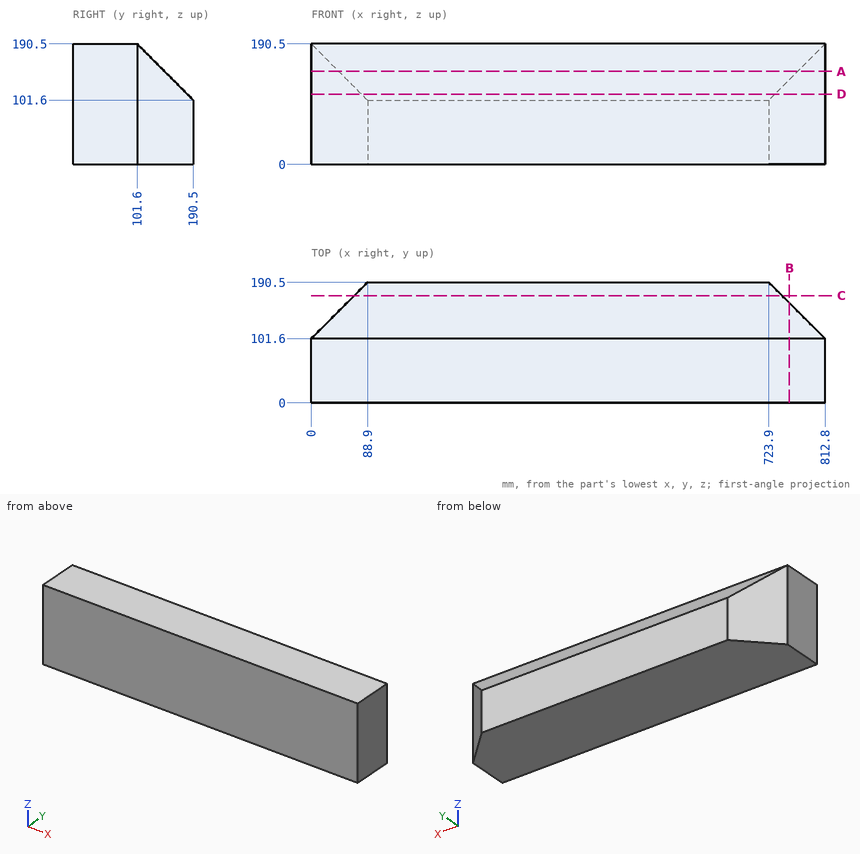
Source: three-view drawing plus pictorial views. Frame: mm from the lowest corner of the part. Round coordinates to 2 decimals unless told otherwise and drop trailing zeros. Loops run counter-clockwise (first coordinate to the right, second up) from the corner with the lowest first, then second, coordinate; pieces in that order, holes last. Notation, with made-up numbers: (-26.75, -20) - (20.25, -20) arc R19 ccw to (20.25, 1) - close; hole circle Ø5 at (81.25, -19). An arc over 180 degrees is marked (long way). Write item = value, one per line. Start each with the question number.
Item 1: Section query C-C on y = 169.5. Output: boundary loops of the cut face in (x, z).
Item 2: Section query A-A on z = 147. Output: boundary loops of the cut face in (x, y).
Item 3: First-contact query: pin 1 Ø1 at (x, z) = (689, 40) entering from -Y; pin 2 Ø1 at (x, z) = (277, 119.5) entering from +Y; pin 3 Ø3 at (x, z) = (348.5, 147) entering from +Y; pin 4 Ø4 at (y, z) = (145, 69.5) entering from -X. Flat tips, straight axial feed; report the tip coordinate or a pass-through.
Item 4: Section query B-B on x = 756.5. Output: boundary loops of the cut face in (y, z).
Item 5: Section query D-D on z = 111. Output: boundary loops of the cut face in (x, y), plus the area to 3 significant figures.
Item 6: Material intervals for line 1 (Z direction, x = 462.5, y = 119.5); line 2 (Z direction, x = 93.5, y = 129.5); line 3 (Y direction, x = 757.5, z = 18), sorted ascending.
Results list:
q1.outline = (67.9, 0) - (744.9, 0) - (744.9, 122.6) - (67.9, 122.6) - close
q2.outline = (0, 0) - (812.8, 0) - (812.8, 101.6) - (769.3, 145.1) - (43.5, 145.1) - (0, 101.6) - close
q3.pin_1 = 0
q3.pin_2 = 173.1
q3.pin_3 = 146.6
q3.pin_4 = 41.4
q4.outline = (0, 0) - (157.9, 0) - (157.9, 134.2) - (101.6, 190.5) - (0, 190.5) - close
q5.outline = (0, 0) - (812.8, 0) - (812.8, 101.6) - (733.3, 181.1) - (79.5, 181.1) - (0, 101.6) - close
q5.area = 141,000 mm²
q6.line_1 = 0 to 172.6
q6.line_2 = 0 to 162.6
q6.line_3 = 0 to 156.9
